from build123d import *

# Parameters (mm, degrees)
SKETCH1_R           = 30
SKETCH1_R_2         = 17.5
BOSS_EXTRUDE1_DEPTH = 7.5
SKETCH2_R           = 1.5
CUT_EXTRUDE1_DEPTH  = 46


with BuildPart() as part:
    # Sketch1 → Boss-Extrude1 (new, symmetric)
    with BuildSketch(Plane(origin=(0, 0, 0), x_dir=(0, 0, -1), z_dir=(1, 0, 0))):
        Circle(SKETCH1_R)
        Circle(SKETCH1_R_2, mode=Mode.SUBTRACT)
    extrude(amount=BOSS_EXTRUDE1_DEPTH, both=True)

    # Sketch2 → Cut-Extrude1 (cut, through all)
    with BuildSketch(Plane(origin=(7.5, 0, 0), x_dir=(0, 0, -1), z_dir=(1, 0, 0))):
        with Locations((0, 20)):
            Circle(SKETCH2_R)
        with Locations((20, 0)):
            Circle(SKETCH2_R)
        with Locations((0, -20)):
            Circle(SKETCH2_R)
        with Locations((-20, 0)):
            Circle(SKETCH2_R)
    extrude(amount=-CUT_EXTRUDE1_DEPTH, mode=Mode.SUBTRACT)


solid = part.part
Design review of the part built by this model. Coordinates are the model's own, in mm. Coordinates: 2 decimals unless noted, no trailing zeros. Loops run counter-clockwise (first coordinate to the right, second up) from the corner with the lowest first, then second, coordinate; pieces in that order, holes last. Notation, with made-up numbers: (23, -24) - (71, -24) arc R7 ccw to (71, -19) - close; hole circle Ø6 at (49, 11.5). An arc over 180 degrees is marked (long way). Use CSV: the item, a comma, the result in double quotes. Start each with the question number.
1. Add section A-A on y = 0. Give the boundary of the cut face in (x, z).
2. To check wall thickness, follow probe 1 along Y at (x, z) = (-4, 0); probe 2 along Z at (x, y) = (0, 1); probe 3 along Y at (x, z) = (0.5, 16). State the ranges of each line that lie inside material, in increasing order.
3. Add section C-C on y = -7. Give the boundary of the cut face in (x, z), plus the area to 3 significant figures.
4. Clearance check with flat-ended pins moving along their axes: pin 1 (3.5 mm diameter, centred on y = 20, z = 0, fed in from -X); pin 2 (2 mm diameter, centred on x = -3.5, z = 20.5, fed in from -Y); pin 3 (2 mm diameter, centred on x = 5.5, y = 21, fed in from -Z); pin 4 (5 mm diameter, centred on x = 6, z = 0.5, fed in from -Y). State where each tip first meets the part, or that it passes through.
5. Mouldability with a two-part tool opening along Z and no side actions: class faces 1 (the cylindrical face through (0.11, 1.32, 29.97)), 2 (the flat face through (-7.5, -13, -13)), 3 (the cylindrical face through (0.11, 0.07, -18.5)) as released by +Z, released by -Z, zero draft, split by the parting line, or undercut.
6. Add section D-D on z = 11. Give the boundary of the cut face in (x, y), plus the area to 3 significant figures.
Resolved:
1,outline,"(-7.5, -30) - (7.5, -30) - (7.5, -21.5) - (-7.5, -21.5) - close; (-7.5, -18.5) - (7.5, -18.5) - (7.5, -17.5) - (-7.5, -17.5) - close; (-7.5, 17.5) - (7.5, 17.5) - (7.5, 18.5) - (-7.5, 18.5) - close; (-7.5, 21.5) - (7.5, 21.5) - (7.5, 30) - (-7.5, 30) - close"
2,probe 1,"-30 to -21.5, -18.5 to -17.5, 17.5 to 18.5, 21.5 to 30"
2,probe 2,"-29.98 to -21.12, -18.88 to -17.47, 17.47 to 18.88, 21.12 to 29.98"
2,probe 3,"-25.38 to -7.09, 7.09 to 25.38"
3,outline,"(-7.5, -29.17) - (7.5, -29.17) - (7.5, -16.04) - (-7.5, -16.04) - close; (-7.5, 16.04) - (7.5, 16.04) - (7.5, 29.17) - (-7.5, 29.17) - close"
3,area,"394 mm2"
4,pin 1,"x = -7.5"
4,pin 2,"y = -22.8"
4,pin 3,"z = -22.36"
4,pin 4,"y = -30"
5,face 1,"split by the parting line"
5,face 2,"zero draft"
5,face 3,"undercut"
6,outline,"(-7.5, -27.91) - (7.5, -27.91) - (7.5, -13.61) - (-7.5, -13.61) - close; (-7.5, 13.61) - (7.5, 13.61) - (7.5, 27.91) - (-7.5, 27.91) - close"
6,area,"429 mm2"
